CAD build for the part. Positions are in the model's coordinates, mm. A direction names the side the tool comes from. Coordinates: 2 decimals unless noted, no trailing zeros. Loops run counter-clockwise (first coordinate to the right, second up) from the corner with the lowest first, then second, coordinate; pieces in that order, holes last.
1) Saw through at B-B, the plane x = -2.5. Write the cut outline in (y, z), and give its area (3 significant figures).
2) Saw through at A-A, the plane z = 9. Write the cut outline in (x, y) (3 decimals).
3) Pin check, flat tips, straight feed: pin 1 Ø5 at (x, y) = (-1, 56) entering from +Z; pin 2 Ø1 at (x, y) = (-3.5, 36) entering from -Z; pin 3 Ø1.5 at (x, y) = (-4.5, 28) entering from +Z. Stop position of each tip, or through.
4) Wall check: line 1 along Y through (x, z) = (0, 3.5) (3 decimals); line 2 along Y through (x, z) = (-5, 8.75); line 3 along Z through (x, y) = (-3.5, 57.5). Give the ranges that are in metal, low to high.
5) Two-plate mould, pull along X, no slides. Class faces 1 (the flat face through (5, 2.54, 5)), 2 (the cylindrical face through (4.176, 1.252, 10.436)), 3 (the cylindrical face through (-0.056, 56.514, 6.28)): +X half, -X half, draft (parallel to the pull), parting line (faces both ways), or undercut.
6) Which spindle directions (+Z, -Z, +X, -X, +Y, -Y) get a long thin tool onto all of the face, cutting with end or side? Do faces 4 (the flat face through (0, 0, 6)), 5 (the cylindrical face through (4.785, 45.115, 7.857)). Say none if no direction does.
7) Saw through at C-C, the plane y = 14.5. Write the cut outline in (x, z), and give its area (3 significant figures).
8) Saw through at D-D, the plane z = 2.5. Write the cut outline in (x, y) (3 decimals).
Autodesk Fusion 360 part; units mm, degrees
sketch "Sketch1" plane through (0, 0, 0) normal (0, 1, 0) x (1, 0, 0)
  circle A0 centre (0, -6.35) radius 5.0165
  dimension "d1" = 10.033
extrude "Extrude1" add sketch "Sketch1" along normal blind 88.9
hole "Hole1" at (0, 55.245, 11.3665) direction (0, 0, -1) diameter 2.54 depth 19.05 tip angle 118
extrude "Extrude2" cut 1 faces at (-0.3721, 0, 4.7198) along direction (0, 1, 0) blind 2.54
sketch "Sketch3" plane through (0, 2.54, 0) normal (0, -1, 0) x (1, 0, 0)
  circle A0 centre (0, 6.35) radius 5.0165
  line L0 (-2.54, 8.89) -> (2.54, 8.89)
  line L1 (2.54, 8.89) -> (2.54, 3.81)
  line L2 (2.54, 3.81) -> (-2.54, 3.81)
  line L3 (-2.54, 3.81) -> (-2.54, 8.89)
extrude "Extrude3" add sketch "Sketch3" along normal blind 2.54 contours L0 L1 L2 L3
extrude "Extrude4" add 1 faces at (0.8467, 0.8467, 8.89) along direction (0, 0, 1) blind 3.302
extrude "Extrude5" add 1 faces at (2.54, 0.8467, 8.8926) along direction (1, 0, 0) blind 3.302
extrude "Extrude6" add 1 faces at (2.5426, 0.8467, 3.81) along direction (0, 0, -1) blind 3.302
extrude "Extrude7" add 1 faces at (-2.54, 0.8467, 4.908) along direction (-1, 0, 0) blind 3.302
fillet "Fillet1" radius 5.842 4 edges at (-5.842, 1.27, 12.192) (5.842, 1.27, 12.192) (5.842, 1.27, 0.508) (-5.842, 1.27, 0.508)
Data:
1. outline: (0, 1.07) - (2.54, 1.07) - (2.54, 2) - (88.9, 2) - (88.9, 10.7) - (2.54, 10.7) - (2.54, 11.63) - (0, 11.63) - close
1. area: 778 mm2
2. outline: (-5.207, 0) - (5.207, 0) - (5.207, 2.54) - (4.259, 2.54) - (4.259, 88.9) - (-4.259, 88.9) - (-4.259, 2.54) - (-5.207, 2.54) - close; hole circle Ø2.54 at (0, 55.245)
3. pin 1: stops at z = 11.37
3. pin 2: stops at z = 2.33
3. pin 3: stops at z = 9.68
4. line 1: y = 0 to 53.975, 56.515 to 88.9
4. line 2: y = 0 to 2.54
4. line 3: z = 2.76 to 9.94
5. face 1: draft
5. face 2: +X half
5. face 3: undercut
6. face 4: +Z, -Z, +X, -X, -Y
6. face 5: +Y
7. outline: circle Ø10.03 at (0, 6.35)
7. area: 79.1 mm2
8. outline: (-4.395, 0) - (4.395, 0) - (4.395, 2.54) - (3.216, 2.54) - (3.216, 88.9) - (-3.216, 88.9) - (-3.216, 2.54) - (-4.395, 2.54) - close; hole circle Ø2.54 at (0, 55.245)
